```python
from build123d import *

# Parameters (mm, degrees)
CROQUIS1_R              = 1.5
SALIENTE_EXTRUIR1_DEPTH = 3
SALIENTE_EXTRUIR2_DEPTH = 8
CROQUIS3_W              = 13
CROQUIS3_H              = 1.7
CORTAR_EXTRUIR1_DEPTH   = 8
CROQUIS5_W              = 3.5
CROQUIS5_H              = 11
CROQUIS5_W_2            = 6.5
SALIENTE_EXTRUIR3_DEPTH = 1.5
SALIENTE_EXTRUIR4_DEPTH = 1.5
REDONDEO1_R             = 2


with BuildPart() as part:
    # Croquis1 → Saliente-Extruir1 (new body)
    with BuildSketch(Plane.XY):
        with BuildLine():
            Line((-75.306602598, 17.959617496), (-75.306602598, -5.318007663))
            Line((-75.306602598, -5.318007663), (-35.306602598, -5.318007663))
            Line((-35.306602598, -5.318007663), (-35.306602598, 17.959617496))
            ThreePointArc((-35.306602598, 17.959617496), (-35.791122177, 19.26473017), (-37.009921692, 19.937490201))
            Line((-37.009921692, 19.937490201), (-73.603283504, 19.937490201))
            ThreePointArc((-73.603283504, 19.937490201), (-74.822083019, 19.26473017), (-75.306602598, 17.959617496))
        make_face()
        with Locations((-71.306602598, 15.681992337)):
            Circle(CROQUIS1_R, mode=Mode.SUBTRACT)
        with Locations((-39.306602598, 15.681992337)):
            Circle(CROQUIS1_R, mode=Mode.SUBTRACT)
    extrude(amount=SALIENTE_EXTRUIR1_DEPTH)

    # Croquis2 → Saliente-Extruir2 (add)
    with BuildSketch(Plane.XY.offset(3)):
        Polygon((-66.706602598, -5.318007663), (-65.206602598, -5.318007663), (-65.206602598, 16.681992337), (-45.406602598, 16.681992337), (-45.406602598, -5.318007663), (-43.906602598, -5.318007663), (-43.906602598, 18.181992337), (-66.706602598, 18.181992337), align=None)
    extrude(amount=SALIENTE_EXTRUIR2_DEPTH)

    # Croquis3 → Cortar-Extruir1 (cut)
    with BuildSketch(Plane.XZ.offset(5.318007663)):
        with Locations((-58.706602598, 2.15)):
            Rectangle(CROQUIS3_W, CROQUIS3_H)
    extrude(amount=-CORTAR_EXTRUIR1_DEPTH, mode=Mode.SUBTRACT)

    # Croquis5 → Saliente-Extruir3 (add)
    with BuildSketch(Plane.XZ.offset(5.318007663)):
        with Locations((-64.956602598, 5.5)):
            Rectangle(CROQUIS5_W, CROQUIS5_H)
        with Locations((-47.156602598, 5.5)):
            Rectangle(CROQUIS5_W_2, CROQUIS5_H)
    extrude(amount=SALIENTE_EXTRUIR3_DEPTH)

    # Croquis6 → Saliente-Extruir4 (add)
    with BuildSketch(Plane.XY.offset(11)):
        Polygon((-63.206602598, -5.318007663), (-63.206602598, -6.818007663), (-66.706602598, -6.818007663), (-66.706602598, 18.181992337), (-43.906602598, 18.181992337), (-43.906602598, -6.818007663), (-50.406602598, -6.818007663), (-50.406602598, -3.318007663), (-47.406602598, -3.318007663), (-47.406602598, 14.681992337), (-63.206602598, 14.681992337), align=None)
    extrude(amount=SALIENTE_EXTRUIR4_DEPTH)

    # Redondeo1
    # the kernel refuses this fillet: 2 mm, written as the material it takes off along each edge
    with BuildSketch(Plane(origin=(-45.906602598, -4.818007663, 10.5), x_dir=(1, 0, 0), z_dir=(0, 0, 1))) as redondeo1_piece_1_section:
        Polygon((0, 0), (REDONDEO1_R * 1.02, 0), (REDONDEO1_R * 1.02, -REDONDEO1_R * 1.02), (0, -REDONDEO1_R * 1.02), align=None)
    redondeo1_piece_1 = extrude(amount=REDONDEO1_R * 1.02, mode=Mode.PRIVATE)
    redondeo1_piece_1 = redondeo1_piece_1 - Plane(origin=(-45.906602598, -4.818007663, 10.5), x_dir=(-0.7071067811865477, 0.7071067811865474, 0), z_dir=(0, 0, 1)) * Sphere(REDONDEO1_R, mode=Mode.PRIVATE)
    add(redondeo1_piece_1, mode=Mode.SUBTRACT)
    with BuildSketch(Plane(origin=(-45.906602598, 16.181992337, 10.5), x_dir=(0, 1, 0), z_dir=(0, 0, 1))) as redondeo1_piece_2_section:
        Polygon((0, 0), (REDONDEO1_R * 1.02, 0), (REDONDEO1_R * 1.02, -REDONDEO1_R * 1.02), (0, -REDONDEO1_R * 1.02), align=None)
    redondeo1_piece_2 = extrude(amount=REDONDEO1_R * 1.02, mode=Mode.PRIVATE)
    redondeo1_piece_2 = redondeo1_piece_2 - Plane(origin=(-45.906602598, 16.181992337, 10.5), x_dir=(-0.7071067811865471, -0.7071067811865477, 0), z_dir=(0, 0, 1)) * Sphere(REDONDEO1_R, mode=Mode.PRIVATE)
    add(redondeo1_piece_2, mode=Mode.SUBTRACT)
    with BuildSketch(Plane(origin=(-64.706602598, 16.181992337, 10.5), x_dir=(0, 1, 0), z_dir=(0, 0, 1))) as redondeo1_piece_3_section:
        Polygon((0, 0), (REDONDEO1_R * 1.02, 0), (REDONDEO1_R * 1.02, REDONDEO1_R * 1.02), (0, REDONDEO1_R * 1.02), align=None)
    redondeo1_piece_3 = extrude(amount=REDONDEO1_R * 1.02, mode=Mode.PRIVATE)
    redondeo1_piece_3 = redondeo1_piece_3 - Plane(origin=(-64.706602598, 16.181992337, 10.5), x_dir=(0.7071067811865477, -0.7071067811865475, 0), z_dir=(0, 0, 1)) * Sphere(REDONDEO1_R, mode=Mode.PRIVATE)
    add(redondeo1_piece_3, mode=Mode.SUBTRACT)
    with BuildSketch(Plane(origin=(-64.706602598, -4.818007663, 10.5), x_dir=(-1, 0, 0), z_dir=(0, 0, 1))) as redondeo1_piece_4_section:
        Polygon((0, 0), (REDONDEO1_R * 1.02, 0), (REDONDEO1_R * 1.02, REDONDEO1_R * 1.02), (0, REDONDEO1_R * 1.02), align=None)
    redondeo1_piece_4 = extrude(amount=REDONDEO1_R * 1.02, mode=Mode.PRIVATE)
    redondeo1_piece_4 = redondeo1_piece_4 - Plane(origin=(-64.706602598, -4.818007663, 10.5), x_dir=(0.7071067811865475, 0.7071067811865475, 0), z_dir=(0, 0, 1)) * Sphere(REDONDEO1_R, mode=Mode.PRIVATE)
    add(redondeo1_piece_4, mode=Mode.SUBTRACT)
    with BuildSketch(Plane(origin=(-35.306602598, -5.318007663, -5), x_dir=(-1, 0, 0), z_dir=(0, 0, 1))) as redondeo1_piece_5:
        with BuildLine():
            CenterArc((REDONDEO1_R, -REDONDEO1_R), REDONDEO1_R, 90, 90)
            Line((0, -REDONDEO1_R), (0, 0))
            Line((0, 0), (REDONDEO1_R, 0))
        make_face()
    extrude(amount=13, mode=Mode.SUBTRACT)
    with BuildSketch(Plane(origin=(-45.906602598, -6.818007663, 12.5), x_dir=(0, 0, -1), z_dir=(-1, 0, 0))) as redondeo1_piece_6:
        with BuildLine():
            CenterArc((REDONDEO1_R, -REDONDEO1_R), REDONDEO1_R, 90, 90)
            Line((0, -REDONDEO1_R), (0, 0))
            Line((0, 0), (REDONDEO1_R, 0))
        make_face()
    extrude(amount=9.5, mode=Mode.SUBTRACT)
    with BuildSketch(Plane(origin=(-43.906602598, 16.181992337, 12.5), x_dir=(-1, 0, 0), z_dir=(0, -1, 0))) as redondeo1_piece_7:
        with BuildLine():
            CenterArc((REDONDEO1_R, REDONDEO1_R), REDONDEO1_R, 180, 90)
            Line((0, REDONDEO1_R), (0, 0))
            Line((0, 0), (REDONDEO1_R, 0))
        make_face()
    extrude(amount=21, mode=Mode.SUBTRACT)
    with BuildSketch(Plane(origin=(-64.706602598, 18.181992337, 12.5), x_dir=(0, -1, 0), z_dir=(1, 0, 0))) as redondeo1_piece_8:
        with BuildLine():
            CenterArc((REDONDEO1_R, REDONDEO1_R), REDONDEO1_R, 180, 90)
            Line((0, REDONDEO1_R), (0, 0))
            Line((0, 0), (REDONDEO1_R, 0))
        make_face()
    extrude(amount=18.8, mode=Mode.SUBTRACT)
    with BuildSketch(Plane(origin=(-75.306602598, -5.318007663, -5), x_dir=(1, 0, 0), z_dir=(0, 0, 1))) as redondeo1_piece_9:
        with BuildLine():
            CenterArc((REDONDEO1_R, REDONDEO1_R), REDONDEO1_R, 180, 90)
            Line((0, REDONDEO1_R), (0, 0))
            Line((0, 0), (REDONDEO1_R, 0))
        make_face()
    extrude(amount=13, mode=Mode.SUBTRACT)
    with BuildSketch(Plane(origin=(-66.706602598, -4.818007663, 12.5), x_dir=(0, 0, -1), z_dir=(0, 1, 0))) as redondeo1_piece_10:
        with BuildLine():
            CenterArc((REDONDEO1_R, -REDONDEO1_R), REDONDEO1_R, 90, 90)
            Line((0, -REDONDEO1_R), (0, 0))
            Line((0, 0), (REDONDEO1_R, 0))
        make_face()
    extrude(amount=21, mode=Mode.SUBTRACT)
    with BuildSketch(Plane(origin=(-58.206602598, -6.818007663, 12.5), x_dir=(0, 0, -1), z_dir=(-1, 0, 0))) as redondeo1_piece_11:
        with BuildLine():
            CenterArc((REDONDEO1_R, -REDONDEO1_R), REDONDEO1_R, 90, 90)
            Line((0, -REDONDEO1_R), (0, 0))
            Line((0, 0), (REDONDEO1_R, 0))
        make_face()
    extrude(amount=6.5, mode=Mode.SUBTRACT)
    with BuildSketch(Plane(origin=(-66.706602598, 18.181992337, 10.5), x_dir=(0, -1, 0), z_dir=(0, 0, -1))) as redondeo1_piece_12:
        with BuildLine():
            CenterArc((REDONDEO1_R, -REDONDEO1_R), REDONDEO1_R, 90, 90)
            Line((0, -REDONDEO1_R), (0, 0))
            Line((0, 0), (REDONDEO1_R, 0))
        make_face()
    extrude(amount=7.5, mode=Mode.SUBTRACT)
    with BuildSketch(Plane(origin=(-43.906602598, 18.181992337, 3), x_dir=(-1, 0, 0), z_dir=(0, 0, 1))) as redondeo1_piece_13:
        with BuildLine():
            CenterArc((REDONDEO1_R, REDONDEO1_R), REDONDEO1_R, 180, 90)
            Line((0, REDONDEO1_R), (0, 0))
            Line((0, 0), (REDONDEO1_R, 0))
        make_face()
    extrude(amount=7.5, mode=Mode.SUBTRACT)
    with BuildSketch(Plane(origin=(-66.706602598, -6.818007663, -5), x_dir=(0, 1, 0), z_dir=(0, 0, 1))) as redondeo1_piece_14_section:
        with BuildLine():
            CenterArc((REDONDEO1_R, -REDONDEO1_R), REDONDEO1_R, 90, 90)
            Line((0, -REDONDEO1_R), (0, 0))
            Line((0, 0), (REDONDEO1_R, 0))
        make_face()
    redondeo1_piece_14 = extrude(amount=15.5, mode=Mode.PRIVATE)
    redondeo1_piece_14 = split(redondeo1_piece_14, bisect_by=Plane(origin=(-66.254561414, -5.318007663, 1.5), z_dir=(0, -1, 0)), keep=Keep.TOP, mode=Mode.PRIVATE)
    add(redondeo1_piece_14, mode=Mode.SUBTRACT)
    with BuildSketch(Plane(origin=(-66.706602598, -6.818007663, -5), x_dir=(0, 1, 0), z_dir=(0, 0, 1))) as redondeo1_piece_15_section:
        with BuildLine():
            CenterArc((REDONDEO1_R, -REDONDEO1_R), REDONDEO1_R, 90, 90)
            Line((0, -REDONDEO1_R), (0, 0))
            Line((0, 0), (REDONDEO1_R, 0))
        make_face()
    redondeo1_piece_15 = extrude(amount=15.5, mode=Mode.PRIVATE)
    redondeo1_piece_15 = split(redondeo1_piece_15, bisect_by=Plane(origin=(-66.687603103, -5.193408024, 3), z_dir=(0, 0, 1)), keep=Keep.TOP, mode=Mode.PRIVATE)
    add(redondeo1_piece_15, mode=Mode.SUBTRACT)
    with BuildSketch(Plane(origin=(-43.906602598, -6.818007663, -5), x_dir=(-1, 0, 0), z_dir=(0, 0, 1))) as redondeo1_piece_16_section:
        with BuildLine():
            CenterArc((REDONDEO1_R, -REDONDEO1_R), REDONDEO1_R, 90, 90)
            Line((0, -REDONDEO1_R), (0, 0))
            Line((0, 0), (REDONDEO1_R, 0))
        make_face()
    redondeo1_piece_16 = extrude(amount=15.5, mode=Mode.PRIVATE)
    redondeo1_piece_16 = split(redondeo1_piece_16, bisect_by=Plane(origin=(-44.358643782, -5.318007663, 1.5), z_dir=(0, -1, 0)), keep=Keep.TOP, mode=Mode.PRIVATE)
    add(redondeo1_piece_16, mode=Mode.SUBTRACT)
    with BuildSketch(Plane(origin=(-43.906602598, -6.818007663, -5), x_dir=(-1, 0, 0), z_dir=(0, 0, 1))) as redondeo1_piece_17_section:
        with BuildLine():
            CenterArc((REDONDEO1_R, -REDONDEO1_R), REDONDEO1_R, 90, 90)
            Line((0, -REDONDEO1_R), (0, 0))
            Line((0, 0), (REDONDEO1_R, 0))
        make_face()
    redondeo1_piece_17 = extrude(amount=15.5, mode=Mode.PRIVATE)
    redondeo1_piece_17 = split(redondeo1_piece_17, bisect_by=Plane(origin=(-43.925602093, -5.193408024, 3), z_dir=(0, 0, 1)), keep=Keep.TOP, mode=Mode.PRIVATE)
    add(redondeo1_piece_17, mode=Mode.SUBTRACT)


solid = part.part
```
CAD build for the part. Positions are in the model's coordinates, mm. A direction names the side the tool comes from. Coordinates: 2 decimals unless noted, no trailing zeros. Order: outer loops, then holes, each group sorted by start corner. A loop starts at its lowest first (then second) coordinate and runs counter-clockwise, first axis right, second up. Notation, with made-up numbers: (-30.5, 60.25) -> (-16.5, 60.25) arc R21 ccw to (-16.5, 89.25) -> close; hole circle Ø4 at (25.5, 36.5). An arc over 180 degrees is marked (long way). Use one line per item in the form item = value. Start each with the question number.
1) Tool access for faces 4 (the flat face through (-55, 18.182, 7)), 5 (the cylindrical face through (-66.136, 17.581, 6.802)), 6 (the flat face through (-70, -5.318, 2)), 7 (the flat face through (-64, -5.318, 6)): list every direction of +Z, -Z, +X, -X, +Y, -Y with a clear straight run to the whole face (end or side of a thin tool).
2) Band-saw the part on B-B on z = 8.75. Give the cut face in (x, y).
3) Drill centre lines: L1, parallel to X at y = 9, z = 3.75; L2, parallel to Z at x = -39.5, y = -5; L3, parallel to Y at x = -46, z = 9.5. Where is each one in solid material? Low to high. Write a range as [from, to].
4) Band-saw the part on D-D on z = 2. Give the cut face in (x, y).
5) Drop flat-ended pins along their axis: pin 1 (5 mm diameter, centred on x = -47.5, y = 10, fed in from +Z); pin 2 (2 mm diameter, centred on y = 14.5, z = 4.5, fed in from +X); pin 3 (1.5 mm diameter, centred on x = -59.5, z = 1.5, fed in from -Y); pin 4 (1.6 mm diameter, centred on x = -48.5, z = 12, fed in from +Y). Give the stop position or say it passes through.
6) Pull direction Y, two halves, no side cores. Call faces 1 (the cylindrical face through (-66.136, -6.217, 5.177)), 2 (the flat face through (-75.307, 7, 1)), 3 (the flat face through (-47.407, 6, 12)): +Y half, -Y half, draft (parallel to the pull), parting line (faces both ways), or undercut.
7) Band-saw the part on A-A on y = 15.25. Give the cut face in (x, z).
8) Band-saw the part on C-C on y = -2.75. Give the cut face in (x, z).
Entries:
q1.face_4 = +Z, +X, -X, +Y
q1.face_5 = +Z, -X, +Y
q1.face_6 = +Z, -Z, -X, -Y
q1.face_7 = none
q2.outline = (-66.71, -4.82) arc R2 ccw to (-64.71, -6.82) -> (-63.21, -6.82) -> (-63.21, -5.32) -> (-65.21, -5.32) -> (-65.21, 16.68) -> (-45.41, 16.68) -> (-45.41, -5.32) -> (-50.41, -5.32) -> (-50.41, -6.82) -> (-45.91, -6.82) arc R2 ccw to (-43.91, -4.82) -> (-43.91, 16.18) arc R2 ccw to (-45.91, 18.18) -> (-64.71, 18.18) arc R2 ccw to (-66.71, 16.18) -> close
q3.L1 = [-66.71, -65.21], [-45.41, -43.91]
q3.L2 = [0, 3]
q3.L3 = [-6.82, -5.32], [16.68, 18.18]
q4.outline = (-75.31, -3.32) arc R2 ccw to (-73.31, -5.32) -> (-66.64, -5.32) arc R2 ccw to (-64.71, -6.82) -> (-63.21, -6.82) -> (-63.21, -5.32) -> (-65.21, -5.32) -> (-65.21, 2.68) -> (-52.21, 2.68) -> (-52.21, -5.32) -> (-50.41, -5.32) -> (-50.41, -6.82) -> (-45.91, -6.82) arc R2 ccw to (-43.97, -5.32) -> (-37.31, -5.32) arc R2 ccw to (-35.31, -3.32) -> (-35.31, 17.96) arc R2 ccw to (-37.01, 19.94) -> (-73.6, 19.94) arc R2 ccw to (-75.31, 17.96) -> close; hole circle Ø3 at (-71.31, 15.68); hole circle Ø3 at (-39.31, 15.68)
q5.pin_1 = 12.5
q5.pin_2 = -43.91
q5.pin_3 = -5.32
q5.pin_4 = 18.06
q6.face_1 = -Y half
q6.face_2 = draft
q6.face_3 = undercut
q7.outline = (-75.31, 0) -> (-72.74, 0) -> (-72.74, 3) -> (-75.31, 3) -> close; (-69.87, 0) -> (-40.74, 0) -> (-40.74, 3) -> (-43.91, 3) -> (-43.91, 10.5) arc R2 ccw to (-45.91, 12.5) -> (-64.71, 12.5) arc R2 ccw to (-66.71, 10.5) -> (-66.71, 3) -> (-69.87, 3) -> close; (-37.87, 0) -> (-35.31, 0) -> (-35.31, 3) -> (-37.87, 3) -> close; hole (-65.21, 3) -> (-45.41, 3) -> (-45.41, 11) -> (-65.21, 11) -> close
q8.outline = (-75.31, 0) -> (-35.31, 0) -> (-35.31, 3) -> (-43.91, 3) -> (-43.91, 10.5) arc R2 ccw to (-45.91, 12.5) -> (-47.41, 12.5) -> (-47.41, 11) -> (-45.41, 11) -> (-45.41, 3) -> (-52.21, 3) -> (-52.21, 1.3) -> (-65.21, 1.3) -> (-65.21, 11) -> (-63.21, 11) -> (-63.21, 12.5) -> (-64.71, 12.5) arc R2 ccw to (-66.71, 10.5) -> (-66.71, 3) -> (-75.31, 3) -> close
